Input: part model. Units: mm. Frame: model coordinates. Round coordinates to 2 decimals unless told otherwise and drop trailing zeros. Loops run counter-clockwise (first coordinate to the right, second up) from the corner with the lowest first, then second, coordinate; pieces in that order, holes last.
1) Ray query, line 1 along X through (y, z) = (-0.75, -180); line 2 along X through (y, z) = (-4.25, -54); line 3 along X through (y, z) = (-4, -420). Return the intervals inside material, ascending.
2) Section A-A, the plane z = 283. Return loops of the section in (x, y).
3) First-contact query: pin 1 (5 mm diameter, centred on x = 0, z = -60, fed in from +Y); pin 2 (7.5 mm diameter, centred on x = 0, z = -300, fed in from +Y); pin 3 (1.5 mm diameter, centred on y = -5.5, z = 193, fed in from -X); pin 4 (4 mm diameter, centred on y = -4, z = 237, fed in from -X). Flat tips, straight axial feed; report the tip coordinate or a pass-through.
from build123d import *

# Parameters (mm, degrees)
BOSS_EXTRUDE1_DEPTH   = 450
SKETCH2_R             = 3
CUT_EXTRUDE1_DEPTH    = 451.451162725
SKETCH3_R             = 4.75
CUT_EXTRUDE2_DEPTH    = 8.5
LPATTERN1_COUNT       = 100
LPATTERN1_PITCH       = 60
MIRROR2_START         = -14.5
MIRROR2_OUTLINE_R     = 4.75
MIRROR2_DEPTH         = 17.5
MIRROR2_2_OUTLINE_W   = 3.5
MIRROR2_2_OUTLINE_H   = 450
MIRROR2_2_OUTLINE_R   = 4.75
MIRROR2_2_OUTLINE_R_2 = 3
MIRROR2_2_DEPTH       = 3.85
MIRROR2_START_2       = -0.65
MIRROR2_3_OUTLINE_W   = 3.5
MIRROR2_3_OUTLINE_H   = 450
MIRROR2_3_DEPTH       = 1.3
MIRROR2_START_3       = -11.024451
MIRROR2_4_OUTLINE_R   = 4.75
MIRROR2_4_OUTLINE_R_2 = 3
MIRROR2_4_DEPTH       = 5.524451
MIRROR2_START_4       = -450
MIRROR2_5_DEPTH       = 450


with BuildPart() as part:
    # Sketch1 → Boss-Extrude1 (new body)
    with BuildSketch(Plane.XY):
        with BuildLine():
            Line((-6.5, -4.15), (-6.5, -7.15))
            Line((-6.5, -7.15), (-10, -10.65))
            Line((-10, -10.65), (-10, -14.5))
            Line((-10, -14.5), (0, -14.5))
            Line((0, -14.5), (0, 3))
            Line((0, 3), (-7.65, 3))
            Line((-7.65, 3), (-8.003553391, 2.646446609))
            ThreePointArc((-8.003553391, 2.646446609), (-8.484745674, 1.484745674), (-9.646446609, 1.003553391))
            Line((-9.646446609, 1.003553391), (-10, 0.65))
            Line((-10, 0.65), (-10, -0.65))
            Line((-10, -0.65), (-9.646446609, -1.003553391))
            ThreePointArc((-9.646446609, -1.003553391), (-8.484745674, -1.484745674), (-8.003553391, -2.646446609))
            Line((-8.003553391, -2.646446609), (-6.5, -4.15))
        make_face()
    boss_extrude1 = extrude(amount=BOSS_EXTRUDE1_DEPTH)

    # Mirror1: Boss-Extrude1 across plane
    add(boss_extrude1.mirror(Plane(origin=(0, 3, 450), x_dir=(0, 0, 1), z_dir=(-1, 0, 0))))

    # Sketch2 → Cut-Extrude1 (cut, through all)
    with BuildSketch(Plane(origin=(0, 3, 0), x_dir=(1, 0, 0), z_dir=(0, 1, 0))):
        Circle(SKETCH2_R)
    cut_extrude1 = extrude(amount=-CUT_EXTRUDE1_DEPTH, mode=Mode.SUBTRACT)

    # Sketch3 → Cut-Extrude2 (cut)
    with BuildSketch(Plane(origin=(0, 3, 0), x_dir=(1, 0, 0), z_dir=(0, 1, 0))):
        Circle(SKETCH3_R)
    cut_extrude2 = extrude(amount=-CUT_EXTRUDE2_DEPTH, mode=Mode.SUBTRACT)

    # LPattern1: Cut-Extrude1, Cut-Extrude2 ×100
    with Locations(*[(0, 0, i * LPATTERN1_PITCH) for i in range(1, LPATTERN1_COUNT)]):
        add(cut_extrude1, mode=Mode.SUBTRACT)
        add(cut_extrude2, mode=Mode.SUBTRACT)

    # Mirror2: read off the stored shape, not the designer's step
    # Mirror2 outline → Mirror2 (add)
    with BuildSketch(Plane(origin=(0, 0, 0), x_dir=(1, 0, 0), z_dir=(0, 1, 0)).offset(MIRROR2_START)):
        with BuildLine():
            ThreePointArc((-4.75, 0), (0, 4.75), (4.75, 0))
            Line((4.75, 0), (6.5, 0))
            Line((6.5, 0), (6.5, 450))
            Line((6.5, 450), (-6.5, 450))
            Line((-6.5, 450), (-6.5, 0))
            Line((-6.5, 0), (-4.75, 0))
        make_face()
        with Locations((0, 60)):
            Circle(MIRROR2_OUTLINE_R, mode=Mode.SUBTRACT)
        with Locations((0, 120)):
            Circle(MIRROR2_OUTLINE_R, mode=Mode.SUBTRACT)
        with Locations((0, 180)):
            Circle(MIRROR2_OUTLINE_R, mode=Mode.SUBTRACT)
        with Locations((0, 240)):
            Circle(MIRROR2_OUTLINE_R, mode=Mode.SUBTRACT)
        with Locations((0, 300)):
            Circle(MIRROR2_OUTLINE_R, mode=Mode.SUBTRACT)
        with Locations((0, 360)):
            Circle(MIRROR2_OUTLINE_R, mode=Mode.SUBTRACT)
        with Locations((0, 420)):
            Circle(MIRROR2_OUTLINE_R, mode=Mode.SUBTRACT)
    extrude(amount=MIRROR2_DEPTH)

    # Mirror2 2 outline → Mirror2 2 (add)
    # profile 1 of 10: a face of its own
    with BuildSketch(Plane(origin=(0, 0, 0), x_dir=(1, 0, 0), z_dir=(0, 1, 0)).offset(MIRROR2_START)):
        with BuildLine():
            ThreePointArc((-3, 0), (0, 3), (3, 0))
            Line((3, 0), (4.75, 0))
            ThreePointArc((4.75, 0), (0, 4.75), (-4.75, 0))
            Line((-4.75, 0), (-3, 0))
        make_face()
    # profile 2 of 10: a face of its own
    with BuildSketch(Plane(origin=(0, 0, 0), x_dir=(1, 0, 0), z_dir=(0, 1, 0)).offset(MIRROR2_START)):
        with Locations((8.25, 225)):
            Rectangle(MIRROR2_2_OUTLINE_W, MIRROR2_2_OUTLINE_H)
    # profile 3 of 10: a face of its own
    with BuildSketch(Plane(origin=(0, 0, 0), x_dir=(1, 0, 0), z_dir=(0, 1, 0)).offset(MIRROR2_START)):
        with Locations((-8.25, 225)):
            Rectangle(MIRROR2_2_OUTLINE_W, MIRROR2_2_OUTLINE_H)
    # profile 4 of 10: a face of its own
    with BuildSketch(Plane(origin=(0, 0, 0), x_dir=(1, 0, 0), z_dir=(0, 1, 0)).offset(MIRROR2_START)):
        with Locations((0, 60)):
            Circle(MIRROR2_2_OUTLINE_R)
        with Locations((0, 60)):
            Circle(MIRROR2_2_OUTLINE_R_2, mode=Mode.SUBTRACT)
    # profile 5 of 10: a face of its own
    with BuildSketch(Plane(origin=(0, 0, 0), x_dir=(1, 0, 0), z_dir=(0, 1, 0)).offset(MIRROR2_START)):
        with Locations((0, 120)):
            Circle(MIRROR2_2_OUTLINE_R)
        with Locations((0, 120)):
            Circle(MIRROR2_2_OUTLINE_R_2, mode=Mode.SUBTRACT)
    # profile 6 of 10: a face of its own
    with BuildSketch(Plane(origin=(0, 0, 0), x_dir=(1, 0, 0), z_dir=(0, 1, 0)).offset(MIRROR2_START)):
        with Locations((0, 180)):
            Circle(MIRROR2_2_OUTLINE_R)
        with Locations((0, 180)):
            Circle(MIRROR2_2_OUTLINE_R_2, mode=Mode.SUBTRACT)
    # profile 7 of 10: a face of its own
    with BuildSketch(Plane(origin=(0, 0, 0), x_dir=(1, 0, 0), z_dir=(0, 1, 0)).offset(MIRROR2_START)):
        with Locations((0, 240)):
            Circle(MIRROR2_2_OUTLINE_R)
        with Locations((0, 240)):
            Circle(MIRROR2_2_OUTLINE_R_2, mode=Mode.SUBTRACT)
    # profile 8 of 10: a face of its own
    with BuildSketch(Plane(origin=(0, 0, 0), x_dir=(1, 0, 0), z_dir=(0, 1, 0)).offset(MIRROR2_START)):
        with Locations((0, 300)):
            Circle(MIRROR2_2_OUTLINE_R)
        with Locations((0, 300)):
            Circle(MIRROR2_2_OUTLINE_R_2, mode=Mode.SUBTRACT)
    # profile 9 of 10: a face of its own
    with BuildSketch(Plane(origin=(0, 0, 0), x_dir=(1, 0, 0), z_dir=(0, 1, 0)).offset(MIRROR2_START)):
        with Locations((0, 360)):
            Circle(MIRROR2_2_OUTLINE_R)
        with Locations((0, 360)):
            Circle(MIRROR2_2_OUTLINE_R_2, mode=Mode.SUBTRACT)
    # profile 10 of 10: a face of its own
    with BuildSketch(Plane(origin=(0, 0, 0), x_dir=(1, 0, 0), z_dir=(0, 1, 0)).offset(MIRROR2_START)):
        with Locations((0, 420)):
            Circle(MIRROR2_2_OUTLINE_R)
        with Locations((0, 420)):
            Circle(MIRROR2_2_OUTLINE_R_2, mode=Mode.SUBTRACT)
    extrude(amount=MIRROR2_2_DEPTH)

    # Mirror2 3 outline → Mirror2 3 (add)
    with BuildSketch(Plane(origin=(0, 0, 0), x_dir=(1, 0, 0), z_dir=(0, 1, 0)).offset(MIRROR2_START_2)):
        with Locations((8.25, 225)):
            Rectangle(MIRROR2_3_OUTLINE_W, MIRROR2_3_OUTLINE_H)
        with Locations((-8.25, 225)):
            Rectangle(MIRROR2_3_OUTLINE_W, MIRROR2_3_OUTLINE_H)
    extrude(amount=MIRROR2_3_DEPTH)

    # Mirror2 4 outline → Mirror2 4 (add)
    # profile 1 of 8: a face of its own
    with BuildSketch(Plane(origin=(0, 0, 0), x_dir=(1, 0, 0), z_dir=(0, 1, 0)).offset(MIRROR2_START_3)):
        with BuildLine():
            ThreePointArc((-3, 0), (0, 3), (3, 0))
            Line((3, 0), (4.75, 0))
            ThreePointArc((4.75, 0), (0, 4.75), (-4.75, 0))
            Line((-4.75, 0), (-3, 0))
        make_face()
    # profile 2 of 8: a face of its own
    with BuildSketch(Plane(origin=(0, 0, 0), x_dir=(1, 0, 0), z_dir=(0, 1, 0)).offset(MIRROR2_START_3)):
        with Locations((0, 60)):
            Circle(MIRROR2_4_OUTLINE_R)
        with Locations((0, 60)):
            Circle(MIRROR2_4_OUTLINE_R_2, mode=Mode.SUBTRACT)
    # profile 3 of 8: a face of its own
    with BuildSketch(Plane(origin=(0, 0, 0), x_dir=(1, 0, 0), z_dir=(0, 1, 0)).offset(MIRROR2_START_3)):
        with Locations((0, 120)):
            Circle(MIRROR2_4_OUTLINE_R)
        with Locations((0, 120)):
            Circle(MIRROR2_4_OUTLINE_R_2, mode=Mode.SUBTRACT)
    # profile 4 of 8: a face of its own
    with BuildSketch(Plane(origin=(0, 0, 0), x_dir=(1, 0, 0), z_dir=(0, 1, 0)).offset(MIRROR2_START_3)):
        with Locations((0, 180)):
            Circle(MIRROR2_4_OUTLINE_R)
        with Locations((0, 180)):
            Circle(MIRROR2_4_OUTLINE_R_2, mode=Mode.SUBTRACT)
    # profile 5 of 8: a face of its own
    with BuildSketch(Plane(origin=(0, 0, 0), x_dir=(1, 0, 0), z_dir=(0, 1, 0)).offset(MIRROR2_START_3)):
        with Locations((0, 240)):
            Circle(MIRROR2_4_OUTLINE_R)
        with Locations((0, 240)):
            Circle(MIRROR2_4_OUTLINE_R_2, mode=Mode.SUBTRACT)
    # profile 6 of 8: a face of its own
    with BuildSketch(Plane(origin=(0, 0, 0), x_dir=(1, 0, 0), z_dir=(0, 1, 0)).offset(MIRROR2_START_3)):
        with Locations((0, 300)):
            Circle(MIRROR2_4_OUTLINE_R)
        with Locations((0, 300)):
            Circle(MIRROR2_4_OUTLINE_R_2, mode=Mode.SUBTRACT)
    # profile 7 of 8: a face of its own
    with BuildSketch(Plane(origin=(0, 0, 0), x_dir=(1, 0, 0), z_dir=(0, 1, 0)).offset(MIRROR2_START_3)):
        with Locations((0, 360)):
            Circle(MIRROR2_4_OUTLINE_R)
        with Locations((0, 360)):
            Circle(MIRROR2_4_OUTLINE_R_2, mode=Mode.SUBTRACT)
    # profile 8 of 8: a face of its own
    with BuildSketch(Plane(origin=(0, 0, 0), x_dir=(1, 0, 0), z_dir=(0, 1, 0)).offset(MIRROR2_START_3)):
        with Locations((0, 420)):
            Circle(MIRROR2_4_OUTLINE_R)
        with Locations((0, 420)):
            Circle(MIRROR2_4_OUTLINE_R_2, mode=Mode.SUBTRACT)
    extrude(amount=MIRROR2_4_DEPTH)

    # Mirror2 5 outline → Mirror2 5 (add)
    with BuildSketch(Plane.XY.offset(MIRROR2_START_4)):
        Polygon((-6.5, -10.65), (-6.5, -7.15), (-10, -10.65), align=None)
        with BuildLine():
            Line((-8.003553391, -2.646446609), (-6.5, -4.15))
            Line((-6.5, -4.15), (-6.5, -0.65))
            Line((-6.5, -0.65), (-10, -0.65))
            Line((-10, -0.65), (-9.646446609, -1.003553391))
            ThreePointArc((-9.646446609, -1.003553391), (-8.484745674, -1.484745674), (-8.003553391, -2.646446609))
        make_face()
        with BuildLine():
            Line((7.65, 3), (6.5, 3))
            Line((6.5, 3), (6.5, 0.65))
            Line((6.5, 0.65), (10, 0.65))
            Line((10, 0.65), (9.646446609, 1.003553391))
            ThreePointArc((9.646446609, 1.003553391), (8.484745674, 1.484745674), (8.003553391, 2.646446609))
            Line((8.003553391, 2.646446609), (7.65, 3))
        make_face()
        with BuildLine():
            Line((-6.5, 3), (-7.65, 3))
            Line((-7.65, 3), (-8.003553391, 2.646446609))
            ThreePointArc((-8.003553391, 2.646446609), (-8.484745674, 1.484745674), (-9.646446609, 1.003553391))
            Line((-9.646446609, 1.003553391), (-10, 0.65))
            Line((-10, 0.65), (-6.5, 0.65))
            Line((-6.5, 0.65), (-6.5, 3))
        make_face()
        with BuildLine():
            Line((6.5, -0.65), (6.5, -4.15))
            Line((6.5, -4.15), (8.003553391, -2.646446609))
            ThreePointArc((8.003553391, -2.646446609), (8.484745674, -1.484745674), (9.646446609, -1.003553391))
            Line((9.646446609, -1.003553391), (10, -0.65))
            Line((10, -0.65), (6.5, -0.65))
        make_face()
        Polygon((10, -10.65), (6.5, -7.15), (6.5, -10.65), align=None)
    extrude(amount=MIRROR2_5_DEPTH)


solid = part.part
Final values:
1. line 1: x = -9.9 to -4.75, 4.75 to 9.9
1. line 2: x = -6.5 to 6.5
1. line 3: x = -6.65 to -4.75, 4.75 to 6.65
2. outline: (-10, -14.5) - (10, -14.5) - (10, -10.65) - (6.5, -7.15) - (6.5, -4.15) - (8, -2.65) arc R1.64 cw to (9.65, -1) - (10, -0.65) - (10, 0.65) - (9.65, 1) arc R1.64 cw to (8, 2.65) - (7.65, 3) - (-7.65, 3) - (-8, 2.65) arc R1.64 cw to (-9.65, 1) - (-10, 0.65) - (-10, -0.65) - (-9.65, -1) arc R1.64 cw to (-8, -2.65) - (-6.5, -4.15) - (-6.5, -7.15) - (-10, -10.65) - close
3. pin 1: passes through
3. pin 2: stops at y = -5.5
3. pin 3: stops at x = -6.5
3. pin 4: stops at x = -8.14
